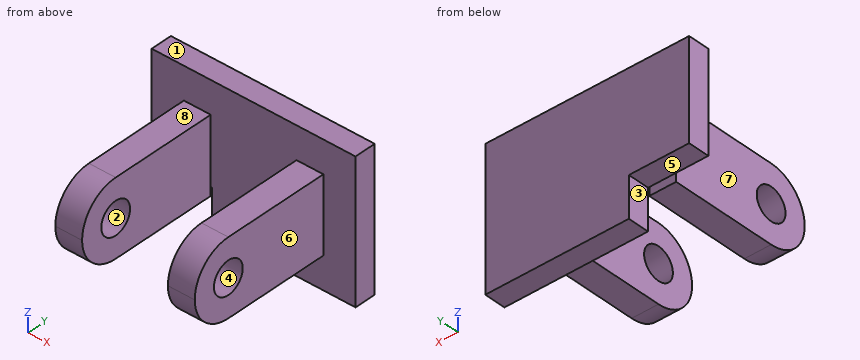
Solid Edge part; units mm, degrees
sketch "Sketch1" plane through (0, 0, 0) normal (0, -1, 0) x (1, 0, 0)
  line L0 (-6.5, -3.5) -> (6.5, -3.5)
  line L1 (6.5, -3.5) -> (6.5, 3.5)
  line L2 (6.5, 3.5) -> (-6.5, 3.5)
  line L3 (-6.5, 3.5) -> (-6.5, -3.5)
extrude "Protrusion1" add sketch "Sketch1" along normal mid plane 13.4
sketch "Sketch2" plane through (0, 6.7, 0) normal (0, 1, 0) x (0, 0, -1)
  line L0 (6.5, 9.5) -> (-6.5, 9.5)
  line L1 (-6.5, 9.5) -> (-6.5, -9.5)
  line L2 (-6.5, -9.5) -> (6.5, -9.5)
  line L3 (6.5, -9.5) -> (6.5, 9.5)
extrude "ExtrudedProtrusion_2" add sketch "Sketch2" along normal blind 2
sketch "Sketch3" plane through (0, 8.7, 0) normal (0, 1, 0) x (1, 0, 0)
  line L0 (-3.8842, 6.5) -> (-3.8842, 2.7306)
  line L1 (-3.8842, 2.7306) -> (-9.5, 2.7306)
  line L2 (-9.5, 2.7306) -> (-9.5, 6.5)
  line L3 (-9.5, 6.5) -> (-3.8842, 6.5)
extrude "Cutout1" cut sketch "Sketch3" against normal up to surface (2 mm away)
fillet "Round_1" radius 3.5 2 edges at (0, -6.7, 3.5) (0, -6.7, -3.5)
hole "Hole_1" at (6.5, -3.2, 0) direction (-1, 0, 0) diameter 3 end up to next
sketch "Sketch4" plane through (0, 1.75, 3.5) normal (0, 0, 1) x (1, 0, 0)
  line L0 (4, 4.95) -> (-4, 4.95)
  line L1 (-4, 4.95) -> (-4, -8.45)
  line L2 (-4, -8.45) -> (4, -8.45)
  line L3 (4, -8.45) -> (4, 4.95)
  dimension "D1" = 4
extrude "Cutout2" cut sketch "Sketch4" against normal up to surface (7 mm away)
properties material "Aluminum, 6061-T6"
CAD build for the part. Positions are in the model's coordinates, mm. Face numbers are marked on the shaded views. A direction names the side the tool comes from. Round coordinates to 2 decimals unless told otherwise and drop trailing zeros. Loops run counter-clockwise (first coordinate to the right, second up) from the corner with the lowest first, then second, coordinate; pieces in that order, holes last. Notation, with made-up numbers: (33, 18) - (79, 18) arc R25 cw to (79, 35) - close; hole circle Ø5 at (77, 8.5). An arc over 180 degrees is marked (long way). Return JSON: item names as keys, results as strings. Group by question number.
Q1. Band-saw the part on D-D on y = -3.5. Give the cut face in (x, z).
Q2. Two-plate mould, pull along Z, no slides. Class the marked faces 1, 2, 3 and 4: +Z half, -Z half, draft (parallel to the pull), parting line (faces both ways), or undercut.
Q3. Band-saw the part on C-C on z = 1.25. Give the cut face in (x, y).
Q4. Drill centre lines: line 1 along Y through (x, z) = (-4.45, 0); line 2 along Z through (x, y) = (5.45, -3.2); line 3 along X through (y, z) = (4.5, -2.5). Where is each one in solid material? Low to high. Write a range as [from, to].
Q5. Flat gauge pins, fed straight in: pin 1 Ø2 at (x, y) = (5.5, 1.5) entering from -Z; pin 2 Ø5.5 at (y, z) = (-0.5, 0) entering from +X; pin 3 Ø4 at (y, z) = (3, 0) entering from -X; pin 4 Ø4 at (x, z) = (-4, -0.5) entering from -Y. Where does each tip first touch, or does it go through?
Q6. Tool access for the marked faces 5, 6, 7 and 8: list every direction of +Z, -Z, +X, -X, +Y, -Y with a clear straight run to the whole face (end or side of a thin tool).
Q7. Band-saw the part on B-B on y = -5.25. Give the cut face in (x, z), plus the area to 3 significant figures.
Solutions:
{
 "1": {"outline": "(-6.5, -3.49) - (-4, -3.49) - (-4, -1.47) - (-6.5, -1.47) - close; (-6.5, 1.47) - (-4, 1.47) - (-4, 3.49) - (-6.5, 3.49) - close; (4, -3.49) - (6.5, -3.49) - (6.5, -1.47) - (4, -1.47) - close; (4, 1.47) - (6.5, 1.47) - (6.5, 3.49) - (4, 3.49) - close"},
 "2": {"face 1": "+Z half", "face 2": "undercut", "face 3": "draft", "face 4": "undercut"},
 "3": {"outline": "(-9.5, 6.7) - (-6.5, 6.7) - (-6.5, -2.37) - (-4, -2.37) - (-4, 6.7) - (4, 6.7) - (4, -2.37) - (6.5, -2.37) - (6.5, 6.7) - (9.5, 6.7) - (9.5, 8.7) - (-9.5, 8.7) - close; (-6.5, -6.47) - (-4, -6.47) - (-4, -4.03) - (-6.5, -4.03) - close; (4, -6.47) - (6.5, -6.47) - (6.5, -4.03) - (4, -4.03) - close"},
 "4": {"line 1": "y = [-6.7, -4.7], [-1.7, 8.7]", "line 2": "z = [-3.5, -1.5], [1.5, 3.5]", "line 3": "x = [-6.5, -4], [4, 6.5]"},
 "5": {"pin 1": "stops at z = -3.5", "pin 2": "stops at x = 6.5", "pin 3": "stops at x = -6.5", "pin 4": "stops at y = -6.7"},
 "6": {"face 5": "-Z, -X, +Y", "face 6": "+Z, -Z, +X, -Y", "face 7": "+Z, -Z, -X, -Y", "face 8": "+Z, +X, -X, -Y"},
 "7": {"outline": "(-6.5, -2.84) - (-4, -2.84) - (-4, 2.84) - (-6.5, 2.84) - close; (4, -2.84) - (6.5, -2.84) - (6.5, 2.84) - (4, 2.84) - close", "area": "28.4 mm^2"}
}
